```python
from build123d import *

# Parameters (mm, degrees)
SKETCH_1_W               = 80
SKETCH_1_H               = 80
SKETCH_1_R               = 25
EXTRUDE_1_DEPTH          = 5
SKETCH_3_R               = 1.5
CUT_EXTRUDE_2_DEPTH      = 5
PATTERN_CIRCULAR_1_COUNT = 4
FILLET_1_R               = 4
SKETCH_7_W               = 30
SKETCH_7_H               = 6
SKETCH_7_R               = 1.5
EXTRUDE_2_DEPTH          = 5
PATTERN_CIRCULAR_2_COUNT = 4


with BuildPart() as part:
    # Sketch 1 → Extrude 1 (new body)
    with BuildSketch(Plane(origin=(0, 0, 0), x_dir=(1, 0, 0), z_dir=(0, 1, 0))):
        Rectangle(SKETCH_1_W, SKETCH_1_H)
        Circle(SKETCH_1_R, mode=Mode.SUBTRACT)
    extrude(amount=EXTRUDE_1_DEPTH)

    # Sketch 3 → Cut-Extrude 2 (cut)
    with BuildSketch(Plane(origin=(0, 0, 0), x_dir=(1, 0, 0), z_dir=(0, 1, 0))):
        with Locations((0, 36)):
            Circle(SKETCH_3_R)
        with Locations((-35.403805922, 35.403805922)):
            Circle(SKETCH_3_R)
    cut_extrude_2 = extrude(amount=CUT_EXTRUDE_2_DEPTH, mode=Mode.SUBTRACT)

    # Pattern Circular 1: Cut-Extrude 2 ×4 about axis
    pattern_circular_1_axis = Axis((0, 0, 0), (0, 1, 0))
    for i in range(1, PATTERN_CIRCULAR_1_COUNT):
        add(cut_extrude_2.rotate(pattern_circular_1_axis, i * 360 / PATTERN_CIRCULAR_1_COUNT), mode=Mode.SUBTRACT)

    # Fillet 1
    fillet_1_edges = [part.edges().sort_by_distance(p)[0] for p in [
        (40, 2.5, 40),
        (-40, 2.5, 40),
        (-40, 2.5, -40),
        (40, 2.5, -40),
    ]]
    fillet(fillet_1_edges, radius=FILLET_1_R)

    # Sketch 7 → Extrude 2 (add)
    with BuildSketch(Plane(origin=(0, 0, 0), x_dir=(1, 0, 0), z_dir=(0, 1, 0))):
        with Locations((0, -43)):
            Rectangle(SKETCH_7_W, SKETCH_7_H)
        with Locations((-7.5, -43)):
            Circle(SKETCH_7_R, mode=Mode.SUBTRACT)
        with Locations((7.5, -43)):
            Circle(SKETCH_7_R, mode=Mode.SUBTRACT)
    extrude_2 = extrude(amount=EXTRUDE_2_DEPTH)

    # Pattern Circular 2: Extrude 2 ×4 about axis
    pattern_circular_2_axis = Axis((0, 0, 0), (0, 1, 0))
    for i in range(1, PATTERN_CIRCULAR_2_COUNT):
        add(extrude_2.rotate(pattern_circular_2_axis, i * 360 / PATTERN_CIRCULAR_2_COUNT))


solid = part.part
```
Part model, mm, in its own coordinate system. A direction names the side the tool comes from. Coordinates: 2 decimals unless noted, no trailing zeros. Order: outer loops, then holes, each group sorted by start corner. A loop starts at its lowest first (then second) coordinate and runs counter-clockwise, first axis right, second up. Notation, with made-up numbers: (-32, 43) -> (-22, 43) arc R12 ccw to (-22, 52) -> close; hole circle Ø2 at (62.25, -35). An arc over 180 degrees is marked (long way). Put each result on its own line as item: value. Start each with the question number.
(1) Band-saw the part on D-D (z = -28.5). Give the cut face in (x, y).
(2) Probe line 1 along X through (y, z) = (3.55, 43); line 2 along X through (y, z) = (1.9, -36); line 3 along Z through (x, y) = (-1, 1.8). List the from-to ranges inside material, lowest first. Write a range as [from, to].
(3) Band-saw the part on B-B (z = -43). Give the cut face in (x, y), then the cut area to 3 significant figures.
(4) Mould opens along Z. For faces 1 (the face through (44.464, 2.465, 7.825)), 2 (the face through (38.797, 2.535, -38.859)), 3 (the face through (15, 2, -43)) say: pulls with the +Z half, pulls with the -Z half, needs draft (parallel to the pull), parting line crosses it, or undercut.
(5) Band-saw the part on C-C (z = 0). Give the cut face in (x, y), then the cut area to 3 significant figures.
(6) Pin check, flat tips, straight feed: pin 1 Ø2.5 at (x, y) = (21, 2) entering from -Z; pin 2 Ø2.5 at (x, z) = (-7.5, -43) entering from +Y; pin 3 Ø2.5 at (y, z) = (2, 42.5) entering from -X; pin 4 Ø1.5 at (x, y) = (42.5, 2) entering from -Z. Stop position of each tip, or through.
(7) Which spindle directions (+Z, -Z, +X, -X, +Y, -Y) get a long thin tool onto all of the face, cutting with end or side? Do faces 4 (the face through (43, 2, -15)), 5 (the face through (40, 2, 26)), 6 (the face through (-40, 2, 26)), 7 (the face through (0, 2, -46)), 8 (the face through (-44.464, 2.465, -7.825)). Say none if no direction does.
(8) Band-saw the part on A-A (x = 0). Give the cut face in (y, z).
Determined:
1. outline: (-40, 0) -> (40, 0) -> (40, 5) -> (-40, 5) -> close
2. line 1: x = [-15, -9], [-6, 6], [9, 15]
2. line 2: x = [-40, -36.78], [-34.03, -1.5], [1.5, 34.03], [36.78, 40]
2. line 3: z = [-46, -37.12], [-34.88, -24.98], [24.98, 34.88], [37.12, 46]
3. outline: (-15, 0) -> (-9, 0) -> (-9, 5) -> (-15, 5) -> close; (-6, 0) -> (6, 0) -> (6, 5) -> (-6, 5) -> close; (9, 0) -> (15, 0) -> (15, 5) -> (9, 5) -> close
3. area: 120 mm²
4. face 1: undercut
4. face 2: pulls with the -Z half
4. face 3: needs draft
5. outline: (-46, 0) -> (-37.5, 0) -> (-37.5, 5) -> (-46, 5) -> close; (-34.5, 0) -> (-25, 0) -> (-25, 5) -> (-34.5, 5) -> close; (25, 0) -> (34.5, 0) -> (34.5, 5) -> (25, 5) -> close; (37.5, 0) -> (46, 0) -> (46, 5) -> (37.5, 5) -> close
5. area: 180 mm²
6. pin 1: stops at z = -40
6. pin 2: passes through
6. pin 3: stops at x = -15
6. pin 4: stops at z = -15
7. face 4: -Z, +X, +Y, -Y
7. face 5: +Z, +X, +Y, -Y
7. face 6: +Z, -X, +Y, -Y
7. face 7: -Z, +X, -X, +Y, -Y
7. face 8: +Y, -Y
8. outline: (0, -46) -> (5, -46) -> (5, -37.5) -> (0, -37.5) -> close; (0, -34.5) -> (5, -34.5) -> (5, -25) -> (0, -25) -> close; (0, 25) -> (5, 25) -> (5, 34.5) -> (0, 34.5) -> close; (0, 37.5) -> (5, 37.5) -> (5, 46) -> (0, 46) -> close
